```python
from build123d import *

# Parameters (mm, degrees)
F1_DEPTH      = 20
F1_DEPTH_BACK = 20
F3_DEPTH      = 2
F5_DEPTH      = 19.5
F5_DEPTH_BACK = 19.5
F6_W          = 0.375
F6_H          = 7.5
F7_DEPTH      = 0.5
F17_DEPTH     = 1
F19_DEPTH     = 1


with BuildPart() as f1:
    # F0 (on Right) → F1 (new body, two sides)
    with BuildSketch(Plane.YZ) as f1_sk:
        Polygon((0, -7), (0, 0), (-6, 0), (-6, -3.75), align=None)
        Polygon((-6, 0), (0, 0), (0, 7), (-6, 3.75), align=None)
    extrude(amount=F1_DEPTH)
    extrude(f1_sk.sketch, amount=-F1_DEPTH_BACK)

    # F2 (on face) → F3 (join)
    with BuildSketch(Plane(origin=(0, 0, 0), x_dir=(-1, 0, 0), z_dir=(0, 1, 0))):
        with BuildLine():
            ThreePointArc((2.75, -4), (-1.9445436483, -2.0554563517), (0, -6.75))
            ThreePointArc((0, -6.75), (1.9445436483, -5.9445436483), (2.75, -4))
        make_face()
    extrude(amount=F3_DEPTH)

    # F4 (on Right) → F5 (cut, two sides)
    with BuildSketch(Plane.YZ) as f5_sk:
        Polygon((-1, 5.8904322458), (-2.7620611939, 4.9370331568), (-6, 3.185080433), (-6, -3.185), (-1, -5.89), (-1, 0), align=None)
    extrude(amount=-F5_DEPTH, mode=Mode.SUBTRACT)
    extrude(f5_sk.sketch, amount=F5_DEPTH_BACK, mode=Mode.SUBTRACT)

    # F6 (on face) → F7 (join)
    with BuildSketch(Plane.XZ.offset(6)):
        with Locations((-0.1875, 0)):
            Rectangle(F6_W, F6_H)
        with Locations((0.1875, 0)):
            Rectangle(F6_W, F6_H)
        with Locations((6.6875, 0)):
            Rectangle(F6_W, F6_H)
        with Locations((6.3125, 0)):
            Rectangle(F6_W, F6_H)
        with Locations((13.1875, 0)):
            Rectangle(F6_W, F6_H)
        with Locations((12.8125, 0)):
            Rectangle(F6_W, F6_H)
        with Locations((19.6875, 0)):
            Rectangle(F6_W, F6_H)
        with Locations((19.3125, 0)):
            Rectangle(F6_W, F6_H)
        with Locations((-6.6875, 0)):
            Rectangle(F6_W, F6_H)
        with Locations((-6.3125, 0)):
            Rectangle(F6_W, F6_H)
        with Locations((-13.1875, 0)):
            Rectangle(F6_W, F6_H)
        with Locations((-12.8125, 0)):
            Rectangle(F6_W, F6_H)
        with Locations((-19.6875, 0)):
            Rectangle(F6_W, F6_H)
        with Locations((-19.3125, 0)):
            Rectangle(F6_W, F6_H)
    extrude(amount=-F7_DEPTH)

    # F9 (on offset) → F10 (revolve)
    with BuildSketch(Plane.XZ.offset(5.75)):
        Polygon((-13.086971221, -3.3170442338), (-19.1837764068, 3.4343508854), (-19.2789044945, 3.353184308), (-13.3750620526, -3.1845304184), (-13.1797424519, -3.4008207144), align=None)
    revolve(axis=Axis((-16.3269832736, -5.75, 0.0843269448), (-0.6702118448, 0, 0.7421698479)))

    # F9 (on offset) → F11 (revolve)
    with BuildSketch(Plane.XZ.offset(5.75)):
        Polygon((-6.586971221, -3.3170442338), (-12.6837764068, 3.4343508854), (-12.8043608498, 3.3254578575), (-12.7513883635, 3.2667979242), (-6.8750620526, -3.1845304184), (-6.6797424519, -3.4008207144), align=None)
    revolve(axis=Axis((-12.7778746067, -5.75, 3.2961278908), (-0.6702118448, 0, 0.7421698479)))

    # F9 (on offset) → F12 (revolve)
    with BuildSketch(Plane.XZ.offset(5.75)):
        Polygon((-6.2765476378, 3.3505744048), (-0.3750620526, -3.1845304184), (-0.1797424519, -3.4008207144), (-0.086971221, -3.3170442338), (-6.1837764068, 3.4343508854), align=None)
    revolve(axis=Axis((-3.3258048452, -5.75, 0.0830219932), (-0.6702118448, 0, 0.7421698479)))

    # F9 (on offset) → F13 (revolve)
    with BuildSketch(Plane.XZ.offset(5.75)):
        Polygon((0.086971221, -3.3170442338), (0.1797424519, -3.4008207144), (0.3750620526, -3.1845304184), (6.2765476378, 3.3505744048), (6.1837764068, 3.4343508854), align=None)
    revolve(axis=Axis((3.3258048452, -5.75, 0.0830219932), (0.6702118448, 0, 0.7421698479)))

    # F9 (on offset) → F14 (revolve)
    with BuildSketch(Plane.XZ.offset(5.75)):
        Polygon((12.7765476378, 3.3505744048), (12.6837764068, 3.4343508854), (6.586971221, -3.3170442338), (6.6797424519, -3.4008207144), (6.8750620526, -3.1845304184), align=None)
    revolve(axis=Axis((9.8258048452, -5.75, 0.0830219932), (0.6702118448, 0, 0.7421698479)))

    # F9 (on offset) → F15 (revolve)
    with BuildSketch(Plane.XZ.offset(5.75)):
        Polygon((19.2765476378, 3.3505744048), (19.1837764068, 3.4343508854), (13.086971221, -3.3170442338), (13.1797424519, -3.4008207144), (13.3750620526, -3.1845304184), align=None)
    revolve(axis=Axis((16.3258048452, -5.75, 0.0830219932), (0.6702118448, 0, 0.7421698479)))

    # F16 (on face) → F17 (cut)
    with BuildSketch(Plane(origin=(0, -2.9315436242, 5.4120805369), x_dir=(1, 0, 0), z_dir=(0, -0.4762831485, 0.8792919665))):
        Polygon((14.25, 2.8339820398), (8.25, 2.8339820398), (7.5, 2.8339820398), (5.5, 2.8339820398), (9.75, -2.7466899922), align=None)
        Polygon((10, -2.9896899922), (19, -2.9896899922), (14.5, 2.5274729855), align=None)
        Polygon((19.5, -2.9896899922), (19.5, 2.8339820398), (14.75, 2.8339820398), align=None)
        Polygon((5.25, 2.5909820398), (1, -2.9896899922), (9.5, -2.9896899922), align=None)
        Polygon((5, 2.8339820398), (0.5, 2.8339820398), (0.5, -2.9896899922), align=None)
        Polygon((-0.5, -2.9896899922), (-0.5, 2.8339820398), (-5, 2.8339820398), align=None)
        Polygon((-1, -2.9896899922), (-5.25, 2.5909820398), (-9.5, -2.9896899922), align=None)
        Polygon((-8.25, 2.8339820398), (-14.25, 2.8339820398), (-9.75, -2.7466899922), (-5.5, 2.8339820398), (-7.5, 2.8339820398), align=None)
        Polygon((-14.5, 2.5274729855), (-19, -2.9896899922), (-10, -2.9896899922), align=None)
        Polygon((-19.5, 2.8339820398), (-19.5, -2.9896899922), (-14.75, 2.8339820398), align=None)
    extrude(amount=-F17_DEPTH, mode=Mode.SUBTRACT)

    # F18 (on face) → F19 (cut)
    with BuildSketch(Plane(origin=(0, 2, 0), x_dir=(-1, 0, 0), z_dir=(0, 1, 0))):
        with BuildLine():
            ThreePointArc((2.5, -4), (1.767766953, -2.232233047), (0, -1.5))
            ThreePointArc((0, -1.5), (-1.767766953, -5.767766953), (2.5, -4))
        make_face()
    extrude(amount=-F19_DEPTH, mode=Mode.SUBTRACT)


solid = f1.part
```
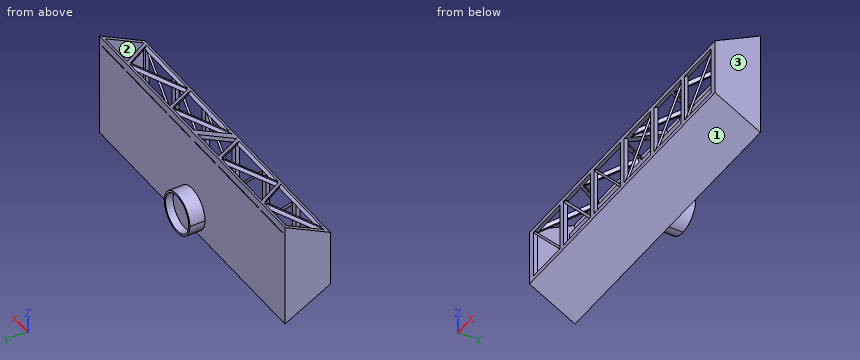
Verification items for the finished model (mm, model axes). Face numbers are marked on the shaded views. Coordinates: 2 decimals unless noted, no trailing zeros. Write each loop counter-clockwise with the first axis right and the second up, starting at its lowest first coordinate (ties: lowest second). Pieces come first, ordered by that corner, then holes. Notation, with made-up numbers: M 27,53 L 42,53 A20 cw 42,72 Z; hole C 86.5,31 d8. An arc over 180 degrees is marked long. Answer as a JSON object with one key per item and string values. Group by question number.
(1) Gauge pin test, flat ends, axial feed: pin 1 (5 mm diameter, centred on x = -8, z = 1, fed in from -Y); pin 2 (6 mm diameter, centred on x = 7.5, z = 3, fed in from +Y); pin 3 (2 mm diameter, centred on x = -1.5, z = -1, fed in from -Y) (3 decimals). Record the tip position at first contact, or that the pin passes through.
(2) Material ranges on line 1 (X direction, y = 1.3, z = -4); line 2 (X direction, y = -2, z = -3); line 3 (Y direction, x = -7.5, z = 4.75), recorded low to high.
(3) Release check for a two-part mould opening along X. For the marked faces 1, 2 and 3 record: +X half, -X half, draft (parallel to the pull), parting line (faces both ways), or undercut.
(4) Cross-section at B-B, the plane y = 0.5. Record the cut outline in (x, z), and give its area (3 significant figures).
Reply:
{
 "1": {"pin 1": "y = -6", "pin 2": "y = 0", "pin 3": "y = -5.875"},
 "2": {"line 1": "-2.75 to -2.5, 2.5 to 2.75", "line 2": "-20 to -19.5, 19.5 to 20", "line 3": "-1 to 0"},
 "3": {"face 1": "draft", "face 2": "undercut", "face 3": "+X half"},
 "4": {"outline": "C 0,-4 d5.5", "area": "23.8 mm²"}
}
